from build123d import *

# Parameters (mm, degrees)
PAD7398_DEPTH   = 38.1
SKETCH8421_W    = 19.05
SKETCH8421_H    = 31.75
PAD7397_DEPTH   = 3.175
POCKET691_DEPTH = 50.801


with BuildPart() as part:
    # Sketch8418 → Pad7398 (new body, symmetric)
    with BuildSketch(Plane.XZ):
        with BuildLine():
            ThreePointArc((0, 14.4145), (-0.892739, 16.569761), (-3.048, 17.4625))
            Line((-3.048, 17.4625), (-50.8, 17.4625))
            Line((-50.8, 17.4625), (-50.8, 14.2875))
            Line((-50.8, 14.2875), (-4.7625, 14.2875))
            ThreePointArc((-3.175, 12.7), (-3.639968, 13.822532), (-4.7625, 14.2875))
            Line((-3.175, 12.7), (-3.175, -12.7))
            ThreePointArc((-4.7625, -14.2875), (-3.639968, -13.822532), (-3.175, -12.7))
            Line((-4.7625, -14.2875), (-50.8, -14.2875))
            Line((-50.8, -14.2875), (-50.8, -17.4625))
            Line((-50.8, -17.4625), (-3.048, -17.4625))
            ThreePointArc((-3.048, -17.4625), (-0.892739, -16.569761), (0, -14.4145))
            Line((0, -14.4145), (0, 14.4145))
        make_face()
    extrude(amount=PAD7398_DEPTH, both=True)

    # Sketch8421 (on DatumPlane) → Pad7397 (join)
    with BuildSketch(Plane.XZ.offset(38.1)):
        with Locations((-15.875, 0)):
            Rectangle(SKETCH8421_W, SKETCH8421_H)
    pad7397 = extrude(amount=-PAD7397_DEPTH)

    # Mirrored017: Pad7397 across XZ
    add(pad7397.mirror(Plane.XZ))

    # Sketch8419 → Pocket691 (cut, through all)
    with BuildSketch(Plane.YZ):
        with BuildLine():
            ThreePointArc((26.19375, 2.38125), (31.75, 7.9375), (26.19375, 13.49375))
            Line((26.19375, 13.49375), (-26.19375, 13.49375))
            ThreePointArc((-26.19375, 13.49375), (-31.75, 7.9375), (-26.19375, 2.38125))
            Line((-26.19375, 2.38125), (26.19375, 2.38125))
        make_face()
        with BuildLine():
            ThreePointArc((26.19375, -13.49375), (31.75, -7.9375), (26.19375, -2.38125))
            Line((26.19375, -2.38125), (-26.19375, -2.38125))
            ThreePointArc((-26.19375, -2.38125), (-31.75, -7.9375), (-26.19375, -13.49375))
            Line((-26.19375, -13.49375), (26.19375, -13.49375))
        make_face()
    extrude(amount=-POCKET691_DEPTH, mode=Mode.SUBTRACT)


solid = part.part
The model under review builds one solid part; all positions refer to its coordinate system, in mm. A direction names the side the tool comes from. Round coordinates to 2 decimals unless told otherwise and drop trailing zeros. Loops run counter-clockwise (first coordinate to the right, second up) from the corner with the lowest first, then second, coordinate; pieces in that order, holes last. Notation, with made-up numbers: (73.25, 16.5) -> (109.25, 16.5) arc R13 cw to (109.25, 33.5) -> close; hole circle Ø10 at (14.25, -30.75). An arc over 180 degrees is marked (long way). One line per question, with ' | ' between items. Start each with the question number.
Item 1: Add section B-B, the plane y = 8.5. Write out the cut boundary in (x, z) (1 decimal).
Item 2: Add section C-C, the plane z = -6. Write out the cut boundary in (x, y) (3 decimals), then the cut area to 3 significant figures.
Item 3: Wall thickness on line 1 along Y through (x, z) = (-7.5, -4.5) (3 decimals); line 2 along Z through (x, y) = (-28, 21.5); line 3 along Z through (x, y) = (-1.5, -20): over which ranges is each line inside the solid? List them lowest first. Write a range as [from, to].
Item 4: For pin 1 (1.7 mm diameter, centred on x = -2, y = -8, fed in from -Z); pin 2 (1 mm diameter, centred on x = -1.5, y = 4, fed in from +Z); pin 3 (8 mm diameter, centred on y = 23.5, z = -4.5, fed in from -X) (3 decimals), all flat-tipped, find the tip position at first contact; note any pin that passes through.
Item 5: Add section D-D, the plane y = 33.5. Write out the cut boundary in (x, z) (1 decimal), then the cut area to 3 significant figures.
Item 6: Add section A-A, the plane x = -42. Write out the cut boundary in (y, z).
Item 7: Machinability: for faces 5 (the face through (0, 0, 1)), 6 (the face through (-1.67, -31.75, -7.82)), 7 (the face through (-25.4, 37, 0)), which of the approach directions +Z, -Z, +X, -X, +Y, -Y give a long, thin tool a straight path to every point of the face, cutting with its end or side? Answer none if there is none.
Item 8: Draft analysis for pull direction X (two halves, no side actions). For faces 1 (the face through (-6.35, 37, 0)), 2 (the face through (-0.917, -0.533, -16.593)), 3 (the face through (-3.175, -3, 0)), 4 (the face through (-50.8, -1, -16)), state which applies: +X half, -X half, draft (parallel to the pull), parting line (faces both ways), or undercut.
Return value:
1) outline: (-50.8, -17.5) -> (-3, -17.5) arc R3 ccw to (0, -14.4) -> (0, -13.5) -> (-3.4, -13.5) arc R1.6 cw to (-4.8, -14.3) -> (-50.8, -14.3) -> close; (-50.8, 14.3) -> (-4.8, 14.3) arc R1.6 cw to (-3.4, 13.5) -> (0, 13.5) -> (0, 14.4) arc R3 ccw to (-3, 17.5) -> (-50.8, 17.5) -> close; (-3.2, -2.4) -> (0, -2.4) -> (0, 2.4) -> (-3.2, 2.4) -> close
2) outline: (-25.4, -38.1) -> (-6.35, -38.1) -> (-6.35, -34.925) -> (-25.4, -34.925) -> close; (-25.4, 34.925) -> (-6.35, 34.925) -> (-6.35, 38.1) -> (-25.4, 38.1) -> close; (-3.175, -38.1) -> (0, -38.1) -> (0, -31.401) -> (-3.175, -31.401) -> close; (-3.175, 31.401) -> (0, 31.401) -> (0, 38.1) -> (-3.175, 38.1) -> close | area: 164 mm2
3) line 1: y = [-38.1, -34.925], [34.925, 38.1] | line 2: z = [-17.46, -14.29], [14.29, 17.46] | line 3: z = [-17.04, -13.49], [-2.38, 2.38], [13.49, 17.04]
4) pin 1: stops at z = -17.46 | pin 2: stops at z = 17.28 | pin 3: stops at x = -3.175
5) outline: (-50.8, -17.5) -> (-3, -17.5) arc R3 ccw to (0, -14.4) -> (0, 14.4) arc R3 ccw to (-3, 17.5) -> (-50.8, 17.5) -> (-50.8, 14.3) -> (-4.8, 14.3) arc R1.6 cw to (-3.2, 12.7) -> (-3.2, -12.7) arc R1.6 cw to (-4.8, -14.3) -> (-50.8, -14.3) -> close | area: 410 mm2
6) outline: (-38.1, -17.46) -> (38.1, -17.46) -> (38.1, -14.29) -> (-38.1, -14.29) -> close; (-38.1, 14.29) -> (38.1, 14.29) -> (38.1, 17.46) -> (-38.1, 17.46) -> close
7) face 5: +Z, -Z, +X, +Y, -Y | face 6: +X, -X | face 7: -X, +Y, -Y
8) face 1: undercut | face 2: +X half | face 3: undercut | face 4: -X half
